from build123d import *

# Parameters (mm, degrees)
SKETCH1_R           = 2.4
BOSS_EXTRUDE1_DEPTH = 71
CUT_EXTRUDE1_START  = -19
CUT_EXTRUDE1_DEPTH  = 19
CHAMFER1_SIZE       = 0.5


with BuildPart() as part:
    # Sketch1 → Boss-Extrude1 (new body)
    with BuildSketch(Plane(origin=(0, 0, 0), x_dir=(1, 0, 0), z_dir=(0, 1, 0))):
        with Locations(Location((0, 0, 0), (0, 0, 270))):
            Circle(SKETCH1_R)
    extrude(amount=BOSS_EXTRUDE1_DEPTH)

    # Sketch2 → Cut-Extrude1 (cut)
    with BuildSketch(Plane(origin=(0, 71, 0), x_dir=(1, 0, 0), z_dir=(0, 1, 0)).offset(CUT_EXTRUDE1_START)):
        with BuildLine():
            Line((1.8734994, 1.5), (1.8734994, -1.5))
            ThreePointArc((1.8734994, -1.5), (2.4, 0), (1.8734994, 1.5))
        make_face()
    extrude(amount=CUT_EXTRUDE1_DEPTH, mode=Mode.SUBTRACT)

    # Chamfer1
    chamfer1_edges = [part.edges().sort_by_distance(p)[0] for p in [
        (0, 0, -2.4),
        (-2.163330765, 71, -1.039230485),
    ]]
    chamfer(chamfer1_edges, length=CHAMFER1_SIZE)


solid = part.part
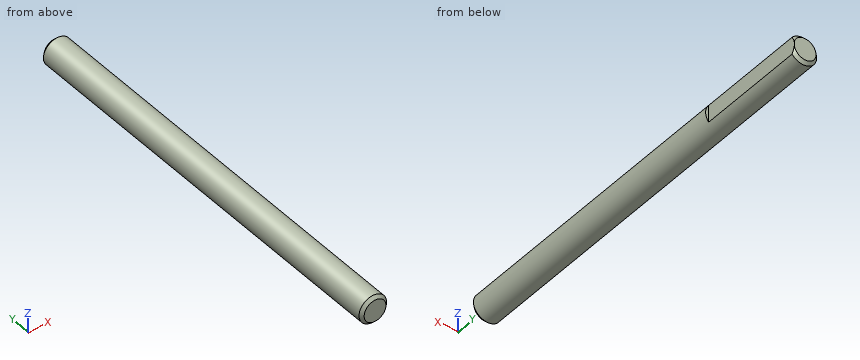
The listing builds one solid part. Answer for the finished solid, in the listing's coordinates (mm). Coordinates: 2 decimals unless noted, no trailing zeros. Write each loop counter-clockwise with the first axis right and the second up, starting at its lowest first coordinate (ties: lowest second). Pieces come first, ordered by that corner, then holes. Notation, with made-up numbers: (38, 52.25) -> (94, 52.25) arc R25 cw to (94, 74.25) -> close; hole circle Ø9 at (12.25, 74). An arc over 180 degrees is marked (long way). One line per question, with ' | ' between items.
1. Given pin 1 Ø2.5 at (y, z) = (66, 0) entering from +X; pin 2 Ø1.5 at (x, y) = (-1.5, 17) entering from -Z, each flat-ended and moving along its own axis, determine where each tip first touches the part or whether it passes through.
Verdict:
pin 1: stops at x = 1.87 | pin 2: stops at z = -2.28
2. Section A-A (y = 53.5) is taken. Determine the outline of the cut face in (x, z).
Verdict:
outline: (1.87, -1.5) -> (1.87, 1.5) arc R2.4 ccw (long way) to start
3. Section B-B (y = 34) is taken. Determine the outline of the cut face in (x, z).
Verdict:
outline: circle Ø4.8 at (0, 0)
4. Straight lines are drawn through the part: line 1 (X direction, y = 41, z = -2.05); line 2 (X direction, y = 6, z = 0.2); line 3 (Y direction, x = 1.65, z = 1.2). For each, find the intervals that lie inside material, in ascending order.
Verdict:
line 1: x = -1.25 to 1.25 | line 2: x = -2.39 to 2.39 | line 3: y = 0.14 to 70.86
